```python
from build123d import *

# Parameters (mm, degrees)
BRIDA_START                = -0.25
BRIDA_BASE1_DEPTH          = 0.25
TALADRO_ROSCADO_M1X0_251_D = 0.75


# Read off the part's stored shape, not the designer's step: Brida base1
with BuildPart() as part:
    # Brida base1 outline → Brida base1 (new body)
    with BuildSketch(Plane.XY.offset(BRIDA_START)):
        with BuildLine():
            ThreePointArc((0.348995339, -0.802388468), (1.480310371, -0.971394868), (2.002599123, -1.989064424))
            Line((2.002599123, -1.989064424), (2.002599123, -2.249894418))
            ThreePointArc((2.002599123, -2.249894418), (2.173526137, -2.836318439), (2.632769916, -3.239064424))
            Line((2.632769916, -3.239064424), (7.459467188, -6.370598579))
            ThreePointArc((7.459467188, -6.370598579), (7.589701514, -6.430586338), (7.731605769, -6.45114585))
            Line((7.731605769, -6.45114585), (8.301442841, -6.45114585))
            ThreePointArc((8.301442841, -6.45114585), (8.430852364, -6.468182936), (8.551442841, -6.518133148))
            Line((8.551442841, -6.518133148), (11.25, -8.07614585))
            ThreePointArc((11.25, -8.07614585), (12.337081426, -6.989064424), (11.25, -5.901982998))
            Line((11.25, -5.901982998), (9.75, -5.901982998))
            ThreePointArc((9.75, -5.901982998), (9.042893219, -5.609089779), (8.75, -4.901982998))
            Line((8.75, -4.901982998), (10.332976724, 0.591177382))
            ThreePointArc((10.332976724, 0.591177382), (10.456141159, 0.802507984), (10.664811028, 0.930128463))
            Line((10.664811028, 0.930128463), (11.123681953, 1.072973914))
            ThreePointArc((11.123681953, 1.072973914), (11.314233531, 1.055602999), (11.436690752, 0.908579595))
            Line((11.436690752, 0.908579595), (11.510997991, 0.669878036))
            Line((11.510997991, 0.669878036), (11.903767414, 0.792146243))
            Line((11.903767414, 0.792146243), (11.866336414, 0.880361426))
            ThreePointArc((11.866336414, 0.880361426), (11.864794565, 1.071948516), (11.999325595, 1.208364763))
            add(Edge.make_bspline(
                [(11.999325595, 1.208364763), (12.49380663, 1.416910388), (12.823037685, 1.541751032), (13.047571984, 1.455257851)],
                knots=[0, 0, 0, 0, 1, 1, 1, 1], degree=3))
            ThreePointArc((13.047571984, 1.455257851), (13.084455869, 1.42899739), (13.111823575, 1.392927439))
            Line((13.111823575, 1.392927439), (13.216225488, 1.200711385))
            Line((13.216225488, 1.200711385), (13.568106318, 1.310251069))
            ThreePointArc((13.568106318, 1.310251069), (13.62691568, 1.359233957), (13.633864046, 1.435454588))
            Line((13.633864046, 1.435454588), (13.624738221, 1.464770016))
            ThreePointArc((13.624738221, 1.464770016), (13.595468937, 1.526984286), (13.550358844, 1.578872492))
            Line((13.550358844, 1.578872492), (12.875597811, 2.16736765))
            ThreePointArc((12.875597811, 2.16736765), (12.424531871, 2.392233856), (11.921080127, 2.368535026))
            Line((11.921080127, 2.368535026), (3.891256423, -0.131130397))
            ThreePointArc((3.891256423, -0.131130397), (3.351888367, -0.146565708), (2.883020599, 0.120490773))
            ThreePointArc((2.883020599, 0.120490773), (1.369312664, 0.946314909), (-0.348995339, 0.802388468))
            ThreePointArc((-0.348995339, 0.802388468), (-0.802388468, -0.348995339), (0.348995339, -0.802388468))
        make_face()
    extrude(amount=BRIDA_BASE1_DEPTH)

    # Taladro roscado M1x0.251 (through all)
    with Locations(Plane.XY):
        with Locations((5.521572875, -1.989064424), (11.25, -6.989064424), (0.75, -1.989064424)):
            Hole(TALADRO_ROSCADO_M1X0_251_D / 2)


solid = part.part
```
Verification items for the finished model (mm, model axes). Coordinates: 2 decimals unless noted, no trailing zeros. Loops run counter-clockwise (first coordinate to the right, second up) from the corner with the lowest first, then second, coordinate; pieces in that order, holes last. Notation, with made-up numbers: (-33.5, -32.75) - (18.5, -32.75) arc R23 ccw to (18.5, 5.25) - close; hole circle Ø6 at (42.25, -24). An arc over 180 degrees is marked (long way). Answer as a JSON object with one key per item and string values.
(1) Cross-section at B-B, the plane x = 0. Record the boundary of the cut face in (y, z) (3 decimals), then the cut area to 3 significant figures.
Response:
{"outline": "(-0.875, -0.25) - (0.916, -0.25) - (0.916, 0) - (-0.875, 0) - close", "area": "0.448 mm²"}
(2) Cross-section at C-C, the plane y = -3. Record the boundary of the cut face in (x, z).
Response:
{"outline": "(2.3, -0.25) - (9.3, -0.25) - (9.3, 0) - (2.3, 0) - close"}
(3) Scan lines: line 1 along Y through (x, z) = (11.25, -0.1); line 2 along Y through (x, z) = (5.5, -0.1); line 3 along Y through (x, z) = (5.75, -0.05). Record each from-to range of solid material in increasing order.
Response:
{"line 1": "y = -8.08 to -7.36, -6.61 to -5.9, 1.08 to 2.16", "line 2": "y = -5.1 to -2.36, -1.61 to 0.37", "line 3": "y = -5.26 to -2.29, -1.69 to 0.45"}
(4) Cross-section at A-A, the plane z = -0.1. Count the separate pieces of the cut face and the enclosed holes in it, then the cut area to 3 significant figures.
Response:
{"separate pieces": "1", "enclosed holes": "2", "area": "55.8 mm²"}
